Input: part model. Units: mm. Frame: model coordinates. A direction names the side the tool comes from. Round coordinates to 2 decimals unless told otherwise and drop trailing zeros. Order: outer loops, then holes, each group sorted by start corner. A loop starts at its lowest first (then second) coordinate and runs counter-clockwise, first axis right, second up. Notation, with made-up numbers: (14, 44.5) -> (39, 44.5) arc R15 ccw to (39, 48.5) -> close; hole circle Ø11 at (71.5, 0). An arc over 180 degrees is marked (long way). Answer as CSV lines item,"result". Start each with the question number.
1) Section query D-D, the plane y = -5. Output: boundary loops of the cut face in (x, z).
2) Line query: L1, parallel to Z at x = 0, y = -0.7; L2, parallel to Z at x = 0, y = 1.4; L3, parallel to X at y = -0.4, z = 0. Output: solid intervals per line, ascending.
3) Section query B-B, the plane y = 2. Output: boundary loops of the cut face in (x, z), and give its area (3 significant figures).
4) Section query A-A, the plane x = 0. State how many separate pieces and enclosed holes the cut face has, and give its area (3 significant figures).
5) Access query for faces 4 (the face through (8, -4, 22)), 5 (the face through (-0.846, 1.479, 8.555)), 6 (the face through (-6, -4, 23)). Directions: +Z, -Z, +X, -X, +Y, -Y. A direction counts if a zero-diameter tool reaches every point of the face in a straight line with its end or side. Return the directions, or none.
6) Section query C-C, the plane z = -12.5. Output: boundary loops of the cut face in (x, y).
7) Mould query, pull axis Z, two halves, no side actions, for faces 1 (the face through (11, -1, 0)), 2 (the face through (3.494, 1.479, -20.481)), 3 (the face through (0, -1, -23.5)). Classes: +Z half, -Z half, draft (parallel to the pull), parting line (faces both ways), or undercut.
8) First-contact query: P1, Ø4.5, axis at x = 0, z = -15, coming from the +Y side; P2, Ø1.2, axis at x = -1.5, y = -4, coming from the +Z side; P3, Ø8, axis at x = 0, z = 15, coming from the -Y side. Flat tips, straight axial feed; report the tip coordinate or a pass-through.
```python
from build123d import *

# Parameters (mm, degrees)
SKETCH2_W           = 22
SKETCH2_H           = 47
SKETCH2_R           = 6.5
BOSS_EXTRUDE1_DEPTH = 3
SKETCH3_W           = 22
SKETCH3_H           = 47
BOSS_EXTRUDE2_DEPTH = 2
BOSS_EXTRUDE3_DEPTH = 4
SKETCH5_5_R         = 2
BOSS_EXTRUDE6_DEPTH = 1
SKETCH5_6_R         = 2
CUT_EXTRUDE1_DEPTH  = 2
SKETCH5_7_W         = 3
SKETCH5_7_H         = 1.5
BOSS_EXTRUDE7_DEPTH = 4


with BuildPart() as part:
    # Sketch2 → Boss-Extrude1 (new body)
    with BuildSketch(Plane(origin=(0, 0, 0), x_dir=(1, 0, 0), z_dir=(0, 1, 0))):
        Rectangle(SKETCH2_W, SKETCH2_H)
        Circle(SKETCH2_R, mode=Mode.SUBTRACT)
        with Locations((0, 15)):
            Circle(SKETCH2_R, mode=Mode.SUBTRACT)
        with Locations((0, -15)):
            Circle(SKETCH2_R, mode=Mode.SUBTRACT)
    extrude(amount=BOSS_EXTRUDE1_DEPTH)

    # Sketch3 → Boss-Extrude2 (add)
    with BuildSketch(Plane.XZ):
        Rectangle(SKETCH3_W, SKETCH3_H)
    extrude(amount=BOSS_EXTRUDE2_DEPTH)

    # Sketch5 → Boss-Extrude3 (add)
    with BuildSketch(Plane(origin=(0, -2, 0), x_dir=(-1, 0, 0), z_dir=(0, -1, 0))):
        Polygon((9, 22), (9, -22), (9, -23.5), (11, -23.5), (11, 23.5), (-11, 23.5), (-11, -23.5), (-9, -23.5), (-9, -22), (-9, 22), align=None)
    extrude(amount=BOSS_EXTRUDE3_DEPTH)

    # Sketch5<5> → Boss-Extrude6 (add)
    with BuildSketch(Plane(origin=(0, -2, 0), x_dir=(-1, 0, 0), z_dir=(0, -1, 0))):
        Circle(SKETCH5_5_R)
    extrude(amount=-BOSS_EXTRUDE6_DEPTH)

    # Sketch5<6> → Cut-Extrude1 (cut)
    with BuildSketch(Plane(origin=(0, -2, 0), x_dir=(-1, 0, 0), z_dir=(0, -1, 0))):
        Circle(SKETCH5_6_R)
        with Locations((0, -15)):
            Circle(SKETCH5_6_R)
        with Locations((0, 15)):
            Circle(SKETCH5_6_R)
    extrude(amount=-CUT_EXTRUDE1_DEPTH, mode=Mode.SUBTRACT)

    # Sketch5<7> → Boss-Extrude7 (add)
    with BuildSketch(Plane(origin=(0, -2, 0), x_dir=(-1, 0, 0), z_dir=(0, -1, 0))):
        with Locations((7.5, -22.75)):
            Rectangle(SKETCH5_7_W, SKETCH5_7_H)
        with Locations((-7.5, -22.75)):
            Rectangle(SKETCH5_7_W, SKETCH5_7_H)
    extrude(amount=BOSS_EXTRUDE7_DEPTH)


solid = part.part
```
Findings:
1,outline,"(-11, -23.5) -> (11, -23.5) -> (11, 23.5) -> (6, 23.5) -> (6, 22) -> (9, 22) -> (9, -22) -> (-9, -22) -> (-9, 22) -> (-6, 22) -> (-6, 23.5) -> (-11, 23.5) -> close"
2,L1,"z = -23.5 to -17, -13 to -2, 2 to 13, 17 to 23.5"
2,L2,"z = -23.5 to -21.5, -8.5 to -6.5, 6.5 to 8.5, 21.5 to 23.5"
2,L3,"x = -11 to -2, 2 to 11"
3,outline,"(-11, -23.5) -> (11, -23.5) -> (11, 23.5) -> (-11, 23.5) -> close; hole circle Ø13 at (0, -15); hole circle Ø13 at (0, 0); hole circle Ø13 at (0, 15)"
3,area,"636 mm^2"
4,separate pieces,"4"
4,enclosed holes,"0"
4,area,"100 mm^2"
5,face 4,"-Y"
5,face 5,"+Y"
5,face 6,"+Z, -Y"
6,outline,"(-11, -6) -> (-9, -6) -> (-9, -2) -> (9, -2) -> (9, -6) -> (11, -6) -> (11, 3) -> (6, 3) -> (6, 0) -> (-6, 0) -> (-6, 3) -> (-11, 3) -> close"
7,face 1,"draft"
7,face 2,"undercut"
7,face 3,"-Z half"
8,P1,"stops at y = 0"
8,P2,"stops at z = -22"
8,P3,"stops at y = -2"
